Verification items for this drawing (mm, ordinates from the low corner). A direction names the side the tool comes from. Coordinates: 2 decimals unless noted, no trailing zeros. Write each loop counter-clockwise with the first axis right and the second up, starting at its lowest first coordinate (ties: lowest second). Pieces come first, ordered by that corner, then holes.
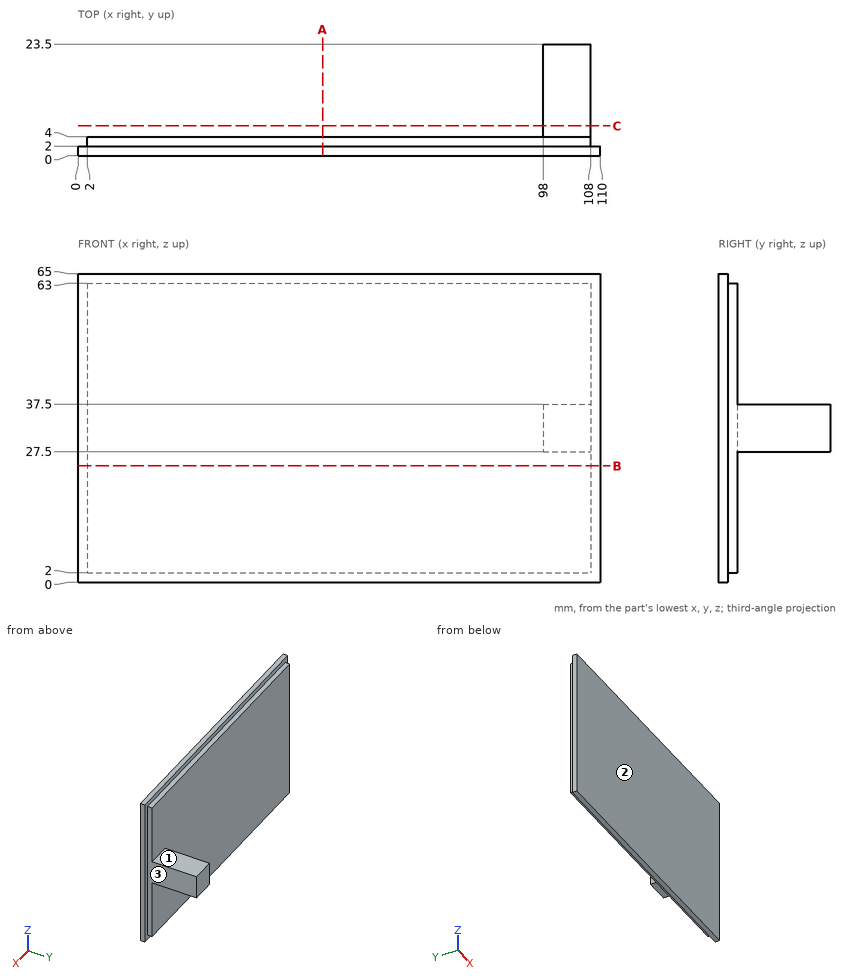
1. Thickness scan on line 1 along Y through (x, z) = (95, 22.5); line 2 along X through (y, z) = (13, 28.5); line 3 along X through (y, z) = (3, 53). Record the ranges inside material, lowest first.
Computed values:
line 1: y = 0 to 4
line 2: x = 98 to 108
line 3: x = 2 to 108
2. Sectioned sample at A-A, the plane x = 51.5. Record the boundary of the cut face in (y, z), and give its area (3 significant figures).
Computed values:
outline: (0, 0) - (2, 0) - (2, 2) - (4, 2) - (4, 63) - (2, 63) - (2, 65) - (0, 65) - close
area: 252 mm2
3. Sectioned sample at B-B, the plane z = 24.5. Record the boundary of the cut face in (x, y), and give its area (3 significant figures).
Computed values:
outline: (0, 0) - (110, 0) - (110, 2) - (108, 2) - (108, 4) - (2, 4) - (2, 2) - (0, 2) - close
area: 432 mm2
4. Access from +Z, -Z, +X, -X, +Y, -Y to the whole of each face (thin tool, end or side, straight path). Record for the marked faces 1, 2 and 3.
Computed values:
face 1: +Z, +X, -X, +Y
face 2: +Z, -Z, +X, -X, -Y
face 3: +Z, -Z, +X, +Y
5. Sectioned sample at C-C, the plane y = 6.25. Record the boundary of the cut face in (x, z).
Computed values:
outline: (98, 27.5) - (108, 27.5) - (108, 37.5) - (98, 37.5) - close
6. Gauge pin test, flat ends, axial feed: pin 1 Ø11 at (x, y) = (101, 10.5) entering from +Z; pin 2 Ø8 at (y, z) = (10, 32) entering from -X; pin 3 Ø12 at (x, y) = (85, 9.5) entering from +Z. Record the tip position at first contact, or that the pin passes through.
Computed values:
pin 1: stops at z = 37.5
pin 2: stops at x = 98
pin 3: stops at z = 63
